Part model, mm, in its own coordinate system. A direction names the side the tool comes from. Coordinates: 2 decimals unless noted, no trailing zeros. Loops run counter-clockwise (first coordinate to the right, second up) from the corner with the lowest first, then second, coordinate; pieces in that order, holes last. Notation, with made-up numbers: (29, 51.5) - (42, 51.5) arc R3 cw to (42, 55.5) - close; hole circle Ø10 at (-11.5, -30.5). An arc over 180 degrees is marked (long way). Use a Markdown table: item, result. Add a question column.
1. Band-saw the part on C-C, the plane y = 15.25. Give the cut face in (x, z).
2. Drop flat-ended pins along their axis: pin 1 (7.5 mm diameter, centred on y = 12, z = -1, fed in from -X); pin 2 (10 mm diameter, centred on y = 15.5, z = -5, fed in from -X); pin 3 (6.5 mm diameter, centred on x = 19, z = 2, fed in from +Y). Give the stop position or say it passes through.
3. 3-axis set-ups, long thin cutter, end or side, ignore diameter. For faces 1 (the cylindrical face through (13.287, 4.288, -0.14)), 2 (the cylindrical face through (29, 10, 0)), 3 (the flat face through (29, 16, 3)): which of +Z, -Z, +X, -X, +Y, -Y reach the whole face in a straight line?
4. Pull direction X, two halves, no side cores. Call faces 4 (the cylindrical face through (-13.313, 4.273, -0.14)), 5 (the flat face through (20, 0, 0)), 6 (the cylindrical face through (-1.5, 9.59, -0.07)): pulls with the +X half, pulls with the -X half, needs draft (parallel to the pull), parting line crosses it, or undercut.
5. Band-saw the part on B-B, the plane x = 0. Give the cut face in (y, z).
6. Band-saw the part on D-D, the plane z = 0. Give the cut face in (x, y), plus the area to 3 significant figures.
7. Band-saw the part on A-A, the plane y = 3.25. Give the cut face in (x, z), plus the area to 3 significant figures.
8. Wall check: probe 1 along Z at (x, y) = (0, 9.7); probe 2 along X at (y, z) = (5.25, -4.25); probe 3 along X at (y, z) = (8, -1). Give the ranges that are in metal, low to high. Write a range as [from, to].
from build123d import *

# Parameters (mm, degrees)
ESTRUSIONE_ESTRUSIONE1_DEPTH = 10
RACCORDO1_R                  = 5
RACCORDO2_R                  = 5
RACCORDO3_R                  = 2
SCHIZZO3_R                   = 2
TAGLIO_ESTRUSIONE1_DEPTH     = 20
SCHIZZO5_R                   = 1.5
TAGLIO_ESTRUSIONE2_DEPTH     = 20
TAGLIO_ESTRUSIONE3_DEPTH     = 20


with BuildPart() as part:
    # Schizzo2 → Estrusione-Estrusione1 (new body, symmetric)
    with BuildSketch(Plane.XY):
        with BuildLine():
            Line((-27.079304388, 0), (-27.079304388, 4))
            Line((-27.079304388, 4), (-13.079304388, 4))
            ThreePointArc((-13.079304388, 4), (0, 12.506273841), (13.079304388, 4))
            Line((13.079304388, 4), (27.079304388, 4))
            Line((27.079304388, 4), (27.079304388, 19))
            Line((27.079304388, 19), (31.079304388, 19))
            Line((31.079304388, 19), (31.079304388, 0))
            Line((31.079304388, 0), (8.496839078, 0))
            ThreePointArc((8.496839078, 0), (0, 6.88360126), (-8.496839078, 0))
            Line((-8.496839078, 0), (-27.079304388, 0))
        make_face()
    extrude(amount=ESTRUSIONE_ESTRUSIONE1_DEPTH, both=True)

    # Raccordo1
    raccordo1_edges = [part.edges().sort_by_distance(p)[0] for p in [
        (29.079304388, 19, -10),
        (29.079304388, 19, 10),
    ]]
    fillet(raccordo1_edges, radius=RACCORDO1_R)

    # Raccordo2
    raccordo2_edges = [part.edges().sort_by_distance(p)[0] for p in [
        (-27.079304388, 2, -10),
        (-27.079304388, 2, 10),
    ]]
    fillet(raccordo2_edges, radius=RACCORDO2_R)

    # Raccordo3
    raccordo3_edges = [part.edges().sort_by_distance(p)[0] for p in [
        (-13.079304388, 4, 0),
        (13.079304388, 4, 0),
    ]]
    fillet(raccordo3_edges, radius=RACCORDO3_R)

    # Schizzo3 → Taglio-Estrusione1 (cut)
    with BuildSketch(Plane(origin=(0, 4, 0), x_dir=(1, 0, 0), z_dir=(0, 1, 0))):
        with Locations((-20.079304388, 5)):
            Circle(SCHIZZO3_R)
    taglio_estrusione1 = extrude(amount=-TAGLIO_ESTRUSIONE1_DEPTH, mode=Mode.SUBTRACT)

    # Specchia1: Taglio-Estrusione1 across plane
    add(taglio_estrusione1.mirror(Plane.XY), mode=Mode.SUBTRACT)

    # Schizzo5 → Taglio-Estrusione2 (cut)
    with BuildSketch(Plane(origin=(0, 0, 0), x_dir=(1, 0, 0), z_dir=(0, 1, 0))):
        Circle(SCHIZZO5_R)
    extrude(amount=TAGLIO_ESTRUSIONE2_DEPTH, mode=Mode.SUBTRACT)

    # Schizzo7 → Taglio-Estrusione3 (cut)
    with BuildSketch(Plane(origin=(31.079304388, 0, 0), x_dir=(0, 0, -1), z_dir=(1, 0, 0))):
        with BuildLine():
            Line((-3, 19), (-3, 13))
            ThreePointArc((-3, 13), (0, 10), (3, 13))
            Line((3, 13), (3, 19))
            Line((3, 19), (-3, 19))
        make_face()
    extrude(amount=-TAGLIO_ESTRUSIONE3_DEPTH, mode=Mode.SUBTRACT)


solid = part.part
Geometry check:
| question | item | result |
|---|---|---|
| 1 | outline | (27.08, -9.84) - (31.08, -9.84) - (31.08, -3) - (27.08, -3) - close; (27.08, 3) - (31.08, 3) - (31.08, 9.84) - (27.08, 9.84) - close |
| 2 | pin 1 | stops at x = -10.18 |
| 2 | pin 2 | stops at x = -7.31 |
| 2 | pin 3 | stops at y = 4 |
| 3 | face 1 | +Z, -Z, +Y |
| 3 | face 2 | +X, +Y |
| 3 | face 3 | +X, -X, +Y |
| 4 | face 4 | pulls with the -X half |
| 4 | face 5 | needs draft |
| 4 | face 6 | undercut |
| 5 | outline | (6.88, -10) - (12.51, -10) - (12.51, -1.5) - (6.88, -1.5) - close; (6.88, 1.5) - (12.51, 1.5) - (12.51, 10) - (6.88, 10) - close |
| 6 | outline | (-27.08, 0) - (-8.5, 0) arc R8.69 cw to (-1.5, 6.75) - (-1.5, 12.43) arc R14.31 ccw to (-12.56, 5.04) arc R2 cw to (-14.32, 4) - (-27.08, 4) - close; (1.5, 6.75) arc R8.69 cw to (8.5, 0) - (31.08, 0) - (31.08, 10) - (27.08, 10) - (27.08, 4) - (14.32, 4) arc R2 cw to (12.56, 5.04) arc R14.31 ccw to (1.5, 12.43) - close |
| 6 | area | 313 mm^2 |
| 7 | outline | (-27.08, -5) arc R5 ccw to (-22.08, -10) - (-7.07, -10) - (-7.07, 10) - (-22.08, 10) arc R5 ccw to (-27.08, 5) - close; (7.07, -10) - (31.08, -10) - (31.08, 10) - (7.07, 10) - close; hole circle Ø4 at (-20.08, -5); hole circle Ø4 at (-20.08, 5) |
| 7 | area | 845 mm^2 |
| 8 | probe 1 | z = [-10, -1.5], [1.5, 10] |
| 8 | probe 2 | x = [-12.45, -5.07], [5.07, 12.45], [27.08, 31.08] |
| 8 | probe 3 | x = [-10.42, -1.12], [1.12, 10.42], [27.08, 31.08] |
